from build123d import *

# Parameters (mm, degrees)
F0_W     = 250
F0_H     = 40
F0_R     = 4.75
F0_R_2   = 3.75
F0_R_3   = 2.75
F0_R_4   = 3.5
F0_R_5   = 4.5
F1_DEPTH = 14
F2_W     = 50
F2_H     = 14
F3_DEPTH = 14


with BuildPart() as f1:
    # F0 (on Top) → F1 (new body)
    with BuildSketch(Plane.XY):
        with Locations((0, -20)):
            Rectangle(F0_W, F0_H)
        with Locations((-100, -20)):
            Circle(F0_R, mode=Mode.SUBTRACT)
        with Locations((-62.5, -20)):
            Circle(F0_R_2, mode=Mode.SUBTRACT)
        with Locations((-30, -20)):
            Circle(F0_R_3, mode=Mode.SUBTRACT)
        with Locations((0, -20)):
            Circle(F0_R_3, mode=Mode.SUBTRACT)
        with Locations((30, -20)):
            Circle(F0_R_4, mode=Mode.SUBTRACT)
        with Locations((62.5, -20)):
            Circle(F0_R_5, mode=Mode.SUBTRACT)
        with Locations((100, -20)):
            Circle(F0_R, mode=Mode.SUBTRACT)
    extrude(amount=F1_DEPTH)

    # F2 (on face) → F3 (join)
    with BuildSketch(Plane(origin=(0, 0, 0), x_dir=(-1, 0, 0), z_dir=(0, 1, 0))):
        with Locations((70, 7)):
            Rectangle(F2_W, F2_H)
        with Locations((-70, 7)):
            Rectangle(F2_W, F2_H)
    extrude(amount=F3_DEPTH)


solid = f1.part
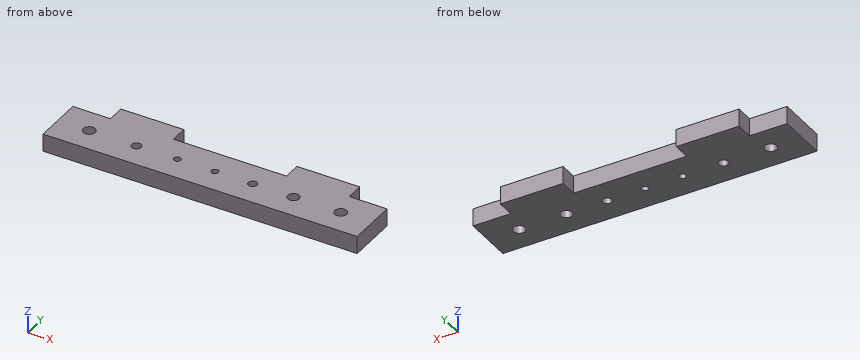
Design review of the part built by this model. Coordinates are the model's own, in mm. Coordinates: 2 decimals unless noted, no trailing zeros. Loops run counter-clockwise (first coordinate to the right, second up) from the corner with the lowest first, then second, coordinate; pieces in that order, holes last. Notation, with made-up numbers: (57.5, -31) - (71.5, -31) arc R19 cw to (71.5, -14) - close; hole circle Ø4 at (37, 87.5). An arc over 180 degrees is marked (long way). Use CSV: the item, a comma, the result in double quotes. Start each with the question number.
1. To check wall thickness, follow probe 1 along Y at (x, z) = (0, 9.25); probe 2 along Y at (x, z) = (-62.5, 10); probe 3 along X at (y, z) = (8.5, 3.25). State the ranges of each line that lie inside material, in increasing order.
2. Add section C-C on z = 7. Give the boundary of the cut face in (x, y).
3. Add section A-A on y = 5. Give the boundary of the cut face in (x, z).
4. Add section B-B on x = -30. Give the boundary of the cut face in (y, z).
5. Clearance check with flat-ended pins moving along their axes: pin 1 (5.5 mm diameter, centred on x = 30, y = -20, fed in from -Z); pin 2 (7 mm diameter, centred on y = 10.5, z = 9.5, fed in from -X); pin 3 (4 mm diameter, centred on x = 116.5, z = 7, fed in from +Y). State where each tip first meets the part, or that it passes through.
6. Add section D-D on y = -20. Count the separate pieces of the cut face and the enclosed holes in it, plus the area to 3 significant figures.
Resolved:
1,probe 1,"-40 to -22.75, -17.25 to 0"
1,probe 2,"-40 to -23.75, -16.25 to 14"
1,probe 3,"-95 to -45, 45 to 95"
2,outline,"(-125, -40) - (125, -40) - (125, 0) - (95, 0) - (95, 14) - (45, 14) - (45, 0) - (-45, 0) - (-45, 14) - (-95, 14) - (-95, 0) - (-125, 0) - close; hole circle Ø9.5 at (-100, -20); hole circle Ø7.5 at (-62.5, -20); hole circle Ø5.5 at (-30, -20); hole circle Ø5.5 at (0, -20); hole circle Ø7 at (30, -20); hole circle Ø9 at (62.5, -20); hole circle Ø9.5 at (100, -20)"
3,outline,"(-95, 0) - (-45, 0) - (-45, 14) - (-95, 14) - close; (45, 0) - (95, 0) - (95, 14) - (45, 14) - close"
4,outline,"(-40, 0) - (-22.75, 0) - (-22.75, 14) - (-40, 14) - close; (-17.25, 0) - (0, 0) - (0, 14) - (-17.25, 14) - close"
5,pin 1,"through"
5,pin 2,"x = -95"
5,pin 3,"y = 0"
6,separate pieces,"8"
6,enclosed holes,"0"
6,area,"2,750 mm2"
